Source: CAD feature listing. Evaluate the final solid. Frame: model axes, mm. A direction names the side the tool comes from. Give positions to 0.01 mm unless a question says otherwise; leave off trailing zeros. Order: outer loops, then holes, each group sorted by start corner. A loop starts at its lowest first (then second) coordinate and runs counter-clockwise, first axis right, second up. Notation, with made-up numbers: M -18.5,5.5 L -12.5,5.5 A23 cw -12.5,21.5 Z; hole C 12,52.5 d7. An arc over 180 degrees is marked long. Answer in a Markdown table with one row per item. Add a question column.
(1) Section query A-A, the plane x = 7. Return loops of the section in (y, z), plus the area to 3 significant figures.
(2) Section query C-C, the plane z = 92. Count the separate pieces of the cut face and the enclosed holes in it, plus the area to 3 significant figures.
(3) Set-up query: faces 5 (the face through (-6, -10, 74)), 6 (the face through (-3.12, -3.77, 73.95)). Return all of +Z, -Z, +X, -X, +Y, -Y with unobstructed straight access to the full face (end or side cutting, diameter ignored); none if empty.
(4) Material intervals for line 1 along Y through (x, z) = (7, 54); line 2 along X through (y, z) = (7.25, 62.5); line 3 along Y through (x, z) = (0, 46), sorted ascending.
(5) Mould query, pull axis Y, two halves, no side actions, for faces 1 (the face through (6, 10, 74)), 2 (the face through (-3.77, 3.12, 73.95)), 3 (the face through (6, -10, 74)), 4 (the face through (-2.4, 0.1, 150)). Classes: pulls with the +Y half, pulls with the -Y half, needs draft (parallel to the pull), parting line crosses it, or undercut.
Autodesk Inventor part; units mm, degrees
ref_plane "YZ Plane" through (0, 0, 0) normal (1, 0, 0) x (0, 1, 0)
ref_plane "XZ Plane" through (0, 0, 0) normal (0, 1, 0) x (-1, 0, 0)
ref_plane "XY Plane" through (0, 0, 0) normal (0, 0, 1) x (1, 0, 0)
sketch "Sketch1" plane through (0, 0, 0) normal (0, 0, 1) x (1, 0, 0)
  line L0 (0, 0) -> (12.2143, 12.2143) construction
  line L1 (0, 0) -> (10, 0) construction
  circle A0 centre (0, 0) radius 2.15
  circle A1 centre (7, 7) radius 2
  circle A2 centre (-7, 7) radius 2
  circle A3 centre (-7, -7) radius 2
  circle A4 centre (7, -7) radius 2
  line L2 (2.95, 10) -> (9.5, 10)
  line L3 (10, 9.5) -> (10, 2.95)
  line L4 (9.7, 2.65) -> (8.9, 2.65)
  line L5 (8.6, 2.95) -> (8.6, 4.2)
  line L6 (4.2, 4.4357) -> (4.2, 8.6)
  line L7 (2.65, 9.7) -> (2.65, 8.9)
  line L8 (2.95, 8.6) -> (4.2, 8.6)
  line L9 (0, 14.2934) -> (0, -14.2934) construction
  arc A5 (2.95, 10) -> (2.65, 9.7) centre (2.95, 9.7) ccw
  arc A6 (2.65, 8.9) -> (2.95, 8.6) centre (2.95, 8.9) ccw
  arc A7 (8.6, 2.95) -> (8.9, 2.65) centre (8.9, 2.95) ccw
  arc A8 (9.7, 2.65) -> (10, 2.95) centre (9.7, 2.95) ccw
  arc A9 (10, 9.5) -> (9.5, 10) centre (9.5, 9.5) ccw
  circle A10 centre (0, 7.1516) radius 5.0016 construction
  circle A11 centre (7.1516, 0) radius 5.0016 construction
  line L10 (8.6, 4.2) -> (4.4357, 4.2)
  line L11 (0, 3) -> (1.9054, 3.3)
  arc A12 (1.9054, 3.3) -> (4.2, 4.4357) centre (0, 10.0357) ccw
  line L12 (3, 0) -> (3.3, 1.9054)
  arc A13 (4.4357, 4.2) -> (3.3, 1.9054) centre (10.0357, 0) ccw
  line L13 (-3, 0) -> (-3.3, 1.9054)
  arc A14 (-3.3, 1.9054) -> (-4.4357, 4.2) centre (-10.0357, 0) ccw
  arc A15 (-4.2, 4.4357) -> (-1.9054, 3.3) centre (0, 10.0357) ccw
  line L14 (0, 3) -> (-1.9054, 3.3)
  line L15 (-4.4357, 4.2) -> (-8.6, 4.2)
  line L16 (-8.6, 2.95) -> (-8.6, 4.2)
  arc A16 (-8.9, 2.65) -> (-8.6, 2.95) centre (-8.9, 2.95) ccw
  line L17 (-9.7, 2.65) -> (-8.9, 2.65)
  arc A17 (-10, 2.95) -> (-9.7, 2.65) centre (-9.7, 2.95) ccw
  line L18 (-10, 2.95) -> (-10, 9.5)
  arc A18 (-9.5, 10) -> (-10, 9.5) centre (-9.5, 9.5) ccw
  line L19 (-9.5, 10) -> (-2.95, 10)
  line L20 (-4.2, 8.6) -> (-4.2, 4.4357)
  line L21 (-2.95, 8.6) -> (-4.2, 8.6)
  arc A19 (-2.95, 8.6) -> (-2.65, 8.9) centre (-2.95, 8.9) ccw
  line L22 (-2.65, 9.7) -> (-2.65, 8.9)
  arc A20 (-2.65, 9.7) -> (-2.95, 10) centre (-2.95, 9.7) ccw
  line L23 (0, -3) -> (-1.9054, -3.3)
  arc A21 (-1.9054, -3.3) -> (-4.2, -4.4357) centre (0, -10.0357) ccw
  arc A22 (-4.4357, -4.2) -> (-3.3, -1.9054) centre (-10.0357, 0) ccw
  line L24 (-3, 0) -> (-3.3, -1.9054)
  line L25 (-4.2, -4.4357) -> (-4.2, -8.6)
  line L26 (-2.95, -8.6) -> (-4.2, -8.6)
  arc A23 (-2.65, -8.9) -> (-2.95, -8.6) centre (-2.95, -8.9) ccw
  line L27 (-2.65, -9.7) -> (-2.65, -8.9)
  arc A24 (-2.95, -10) -> (-2.65, -9.7) centre (-2.95, -9.7) ccw
  line L28 (-2.95, -10) -> (-9.5, -10)
  arc A25 (-10, -9.5) -> (-9.5, -10) centre (-9.5, -9.5) ccw
  line L29 (-10, -9.5) -> (-10, -2.95)
  line L30 (-8.6, -4.2) -> (-4.4357, -4.2)
  line L31 (-8.6, -2.95) -> (-8.6, -4.2)
  arc A26 (-8.6, -2.95) -> (-8.9, -2.65) centre (-8.9, -2.95) ccw
  line L32 (-9.7, -2.65) -> (-8.9, -2.65)
  arc A27 (-9.7, -2.65) -> (-10, -2.95) centre (-9.7, -2.95) ccw
  line L33 (3, 0) -> (3.3, -1.9054)
  arc A28 (3.3, -1.9054) -> (4.4357, -4.2) centre (10.0357, 0) ccw
  arc A29 (4.2, -4.4357) -> (1.9054, -3.3) centre (0, -10.0357) ccw
  line L34 (0, -3) -> (1.9054, -3.3)
  line L35 (4.4357, -4.2) -> (8.6, -4.2)
  line L36 (8.6, -2.95) -> (8.6, -4.2)
  arc A30 (8.9, -2.65) -> (8.6, -2.95) centre (8.9, -2.95) ccw
  line L37 (9.7, -2.65) -> (8.9, -2.65)
  arc A31 (10, -2.95) -> (9.7, -2.65) centre (9.7, -2.95) ccw
  line L38 (10, -2.95) -> (10, -9.5)
  arc A32 (9.5, -10) -> (10, -9.5) centre (9.5, -9.5) ccw
  line L39 (9.5, -10) -> (2.95, -10)
  line L40 (4.2, -8.6) -> (4.2, -4.4357)
  line L41 (2.95, -8.6) -> (4.2, -8.6)
  arc A33 (2.95, -8.6) -> (2.65, -8.9) centre (2.95, -8.9) ccw
  line L42 (2.65, -9.7) -> (2.65, -8.9)
  arc A34 (2.65, -9.7) -> (2.95, -10) centre (2.95, -9.7) ccw
  point P0 (10, 2.65)
  point P1 (8.6, 2.65)
  point P2 (-2.65, 10)
  point P3 (-2.65, 8.6)
  point P4 (-10, -2.65)
  point P5 (-8.6, -2.65)
  point P6 (2.65, -10)
  point P7 (2.65, -8.6)
  dimension "d1" = 45
  dimension "d2" = 4.3
  dimension "d3" = 4
  dimension "d6" = 360
  dimension "d9" = 2.65
  dimension "d10" = 4.2
  dimension "d11" = 1.4
  dimension "d12" = 7
  dimension "d13" = 10
  dimension "d14" = 10
  dimension "d15" = 1.4
  dimension "d16" = 2.65
  dimension "d18" = 0.3
  dimension "d19" = 0.5
  dimension "d22" = 4.2
  dimension "d24" = 6.7
  dimension "d25" = 0.3
  dimension "d26" = 7
  dimension "d27" = 6.7
  dimension "d28" = 0.3
  dimension "d29" = 7
  dimension "d32" = 360
extrude "Extrusion1" add sketch "Sketch1" along normal blind 150
sketch "Sketch2" plane through (2.95, 10, 150) normal (0, 1, 0) x (1, 0, 0)
  line L0 (-2.95, 150) -> (-2.95, 0)
  circle A0 centre (-2.95, 6) radius 2.15
  dimension "d36" = 4.3
  dimension "d37" = 6
extrude "Extrusion2" cut sketch "Sketch2" against normal blind 10
ref_plane "Work Plane1" through (0, 0, 75) normal (0, 0, 1) x (1, 0, 0)
properties part number "Aluminum_Profile_2020"
Values follow:
| question | item | result |
|---|---|---|
| 1 | outline | M -10,0 L -9,0 L -9,150 L -10,150 Z; M -5,0 L -4.2,0 L -4.2,150 L -5,150 Z; M 4.2,0 L 5,0 L 5,150 L 4.2,150 Z; M 9,0 L 10,0 L 10,150 L 9,150 Z |
| 1 | area | 540 mm² |
| 2 | separate pieces | 1 |
| 2 | enclosed holes | 5 |
| 2 | area | 133 mm² |
| 3 | face 5 | +Z, -Z, +X, -X, -Y |
| 3 | face 6 | +Z, -Z |
| 4 | line 1 | y = -10 to -9, -5 to -4.2, 4.2 to 5, 9 to 10 |
| 4 | line 2 | x = -10 to -8.98, -5.02 to -4.2, 4.2 to 5.02, 8.98 to 10 |
| 4 | line 3 | y = -3 to -2.15, 2.15 to 3 |
| 5 | face 1 | pulls with the +Y half |
| 5 | face 2 | undercut |
| 5 | face 3 | pulls with the -Y half |
| 5 | face 4 | needs draft |
